Part model, mm, in its own coordinate system. A direction names the side the tool comes from. Give positions to 0.01 mm unless a question says otherwise; leave off trailing zeros. Loops run counter-clockwise (first coordinate to the right, second up) from the corner with the lowest first, then second, coordinate; pieces in that order, holes last. Notation, with made-up numbers: M 76,80 L 107,80 A27 ccw 107,110 Z; hole C 19,22.5 d8. An arc over 180 degrees is marked long. Put each result on its own line as item: value. Start each with the question number.
```python
from build123d import *

# Parameters (mm, degrees)
F0_R          = 12
F1_DEPTH      = 12
F1_DEPTH_BACK = 12
F2_DEPTH      = 7
F2_DEPTH_BACK = 7
F3_DEPTH      = 28
F3_DEPTH_BACK = 28


with BuildPart() as f1:
    # F0 (on Front) → F1 (new body, two sides)
    with BuildSketch(Plane.XZ) as f1_sk:
        with BuildLine():
            ThreePointArc((-29.435681, 0), (-43.577817, -34.142136), (-9.435681, -20))
            ThreePointArc((-9.435681, -20), (-15.293546, -5.857864), (-29.435681, 0))
        make_face()
        with Locations((-29.435681, -20)):
            Circle(F0_R, mode=Mode.SUBTRACT)
    extrude(amount=F1_DEPTH)
    extrude(f1_sk.sketch, amount=-F1_DEPTH_BACK)

    # F0 (on Front) → F2 (join, two sides)
    with BuildSketch(Plane.XZ) as f2_sk:
        with BuildLine():
            ThreePointArc((-29.435681, 0), (-15.293546, -5.857864), (-9.435681, -20))
            Line((-9.435681, -20), (66.069421, -20))
            ThreePointArc((66.069421, -20), (55.894649, 0.20271), (60.201199, 22.40922))
            Line((60.201199, 22.40922), (-29.435681, 0))
        make_face()
    extrude(amount=F2_DEPTH)
    extrude(f2_sk.sketch, amount=-F2_DEPTH_BACK)

    # F0 (on Front) → F3 (join, two sides)
    with BuildSketch(Plane.XZ) as f3_sk:
        with BuildLine():
            ThreePointArc((60.201199, 22.40922), (55.894649, 0.20271), (66.069421, -20))
            ThreePointArc((66.069421, -20), (104.123054, -27.267022), (125.564319, 5))
            ThreePointArc((125.564319, 5), (99.572393, 38.82092), (60.201199, 22.40922))
        make_face()
        with BuildLine():
            ThreePointArc((115.564319, 5), (108.241988, -12.67767), (90.564319, -20))
            ThreePointArc((90.564319, -20), (74.752931, -14.364917), (66.069421, 0))
            Line((66.069421, 0), (61.564319, 0))
            Line((61.564319, 0), (61.564319, 5))
            Line((61.564319, 5), (61.564319, 10))
            Line((61.564319, 10), (66.069421, 10))
            ThreePointArc((66.069421, 10), (74.752931, 24.364917), (90.564319, 30))
            ThreePointArc((90.564319, 30), (108.241988, 22.67767), (115.564319, 5))
        make_face(mode=Mode.SUBTRACT)
    extrude(amount=F3_DEPTH)
    extrude(f3_sk.sketch, amount=-F3_DEPTH_BACK)


solid = f1.part
```
1) Pin check, flat tips, straight feed: pin 1 Ø8 at (x, z) = (-28.5, -6.5) entering from -Y; pin 2 Ø1 at (y, z) = (18.5, -20) entering from +X; pin 3 Ø3 at (y, z) = (-22.5, 3) entering from -X; pin 4 Ø11 at (y, z) = (-12, 5.5) entering from +X. Stop position of each tip, or through.
2) Mould opens along X. For faces 4 (the flat face through (28, 7, -3)), 5 (the flat face through (16.01, 0.1, 11.36)), 6 (the flat face through (66.7, -28, 13.3)) say: +X half, -X half, draft (parallel to the pull), parting line (faces both ways), or undercut.
3) Band-saw the part on C-C on z = -27. Give the cut face in (x, y).
4) Wall check: L1, parallel to Y at x = 37, z = -17.5; L2, parallel to X at y = 19, z = 17; L3, parallel to X at y = 8, z = 1 (3 decimals). Give the ranges that are in metal, low to high.
5) Band-saw the part on B-B on x = 100. Give the cut face in (y, z), then the cut area to 3 significant figures.
6) Band-saw the part on A-A on y = 4. Give the cut face in (x, z).
7) Band-saw the part on D-D on z = -15. Give the cut face in (x, y), then the cut area to 3 significant figures.
8) Which spindle directions (+Z, -Z, +X, -X, +Y, -Y) get a long thin tool onto all of the face, cutting with end or side? Do faces 1 (the flat face through (64, 0, 0)), 2 (the flat face through (28, 0, -20)), 3 (the flat face through (-21, 12, -29)). Say none if no direction does.
Evaluation:
1. pin 1: y = -12
1. pin 2: x = 115.56
1. pin 3: x = 55.57
1. pin 4: x = 125.56
2. face 4: undercut
2. face 5: -X half
2. face 6: draft
3. outline: M -48.17,-12 L -39.18,-12 L -39.18,12 L -48.17,12 Z; M -19.69,-12 L -10.7,-12 L -10.7,12 L -19.69,12 Z; M 76.39,-28 L 104.74,-28 L 104.74,28 L 76.39,28 Z
4. L1: -7 to 7
4. L2: 57.69 to 68.63, 112.5 to 123.44
4. L3: 55.794 to 61.564, 115.242 to 125.335
5. outline: M -28,-28.7 L 28,-28.7 L 28,-18.15 L -28,-18.15 Z; M -28,28.15 L 28,28.15 L 28,38.7 L -28,38.7 Z
5. area: 1,180 mm2
6. outline: M -29.44,0 A20 ccw long -9.44,-20 L 66.07,-20 A35 ccw long 60.2,22.41 Z; hole C -29.44,-20 d24; hole M 61.56,0 L 66.07,0 A25 ccw 90.56,-20 A25 ccw 90.56,30 A25 ccw 66.07,10 L 61.56,10 Z
7. outline: M -48.8,-12 L -40.34,-12 L -40.34,12 L -48.8,12 Z; M -18.53,-12 L -10.07,-12 L -10.07,-7 L 61.84,-7 L 61.84,-28 L 75.56,-28 L 75.56,28 L 61.84,28 L 61.84,7 L -10.07,7 L -10.07,12 L -18.53,12 Z; M 105.56,-28 L 119.29,-28 L 119.29,28 L 105.56,28 Z
7. area: 2,950 mm2
8. face 1: +Y, -Y
8. face 2: -Z, +Y, -Y
8. face 3: +Z, -Z, -X, +Y
